Part model, mm, in its own coordinate system. Round coordinates to 2 decimals unless told otherwise and drop trailing zeros. Loops run counter-clockwise (first coordinate to the right, second up) from the corner with the lowest first, then second, coordinate; pieces in that order, holes last. Notation, with made-up numbers: (-19.5, 60) - (23.5, 60) arc R11 cw to (23.5, 79) - close; hole circle Ø9 at (8.25, 29). An arc over 180 degrees is marked (long way). Write each question's results on one line, items separated by ' | '. Start each with the question number.
(1) Cut at A-A, the plane z = 288. List the corners of the cut face in (x, y) (3 decimals).
(2) Cut at B-B, the plane x = -4. List the corners of the cut face in (y, z) (3 decimals).
(3) Flat gauge pin, fed straight in: P1, Ø4, axis at y = 25.4, z = 25.4, coming from the +X side. Where does the tip first touch, or does it go through?
(4) Drill centre lines: L1, parallel to Y at x = 10.65, z = 25.4; L2, parallel to X at y = 15, z = 79.5 (3 decimals); L3, parallel to Y at x = 4.25, z = 391.5 (3 decimals). Where is each one in solid material? Low to high.
Autodesk Inventor part; units mm, degrees
ref_plane "Start Plane" through (0, 0, -12.7) normal (0, 0, 1) x (1, 0, 0)
ref_plane "End Plane" through (0, 0, 749.3) normal (0, 0, 1) x (1, 0, 0)
ref_plane "Work Plane6" through (609.6, 0, -12.7) normal (0, 0, -1) x (-1, 0, 0)
ref_plane "Start Plane" through (0, 0, -12.7) normal (0, 0, 1) x (1, 0, 0)
ref_plane "End Plane" through (0, 0, 749.3) normal (0, 0, 1) x (1, 0, 0)
sketch "Sketch" plane through (0, 0, 0) normal (0, 0, 1) x (1, 0, 0)
  line L0 (-12.7, -38.1) -> (12.7, -38.1)
  line L1 (12.7, -38.1) -> (12.7, 38.1)
  line L2 (12.7, 38.1) -> (-12.7, 38.1)
  line L3 (-12.7, 38.1) -> (-12.7, -38.1)
  line L4 (-12.7, -38.1) -> (12.7, 38.1) construction
  line L5 (12.7, -38.1) -> (-12.7, 38.1) construction
  line L6 (-9.525, -34.925) -> (9.525, -34.925)
  line L7 (9.525, -34.925) -> (9.525, 34.925)
  line L8 (9.525, 34.925) -> (-9.525, 34.925)
  line L9 (-9.525, 34.925) -> (-9.525, -34.925)
  line L10 (-9.525, -34.925) -> (9.525, 34.925) construction
  line L11 (9.525, -34.925) -> (-9.525, 34.925) construction
  point P0 (0, 0)
  dimension "d0" = 25.4
  dimension "d1" = 76.2
  dimension "d2" = 3.175
  dimension "d3" = 3.175
extrude "Body" add sketch "Sketch" along normal up to surface (762 mm away) from surface at -12.7
sketch "Sketch6" plane through (0, 0, 0) normal (0, 0, 1) x (1, 0, 0)
  line L0 (0, 0) -> (10, 0)
ref_plane "Work Plane5" through (0, 0, 0) normal (0, -1, 0) x (1, 0, 0)
sketch "Sketch7" plane through (0, 0, 0) normal (0, -1, 0) x (1, 0, 0)
  line L0 (-2, -12.7) -> (12, -12.7)
  line L1 (-2, 749.3) -> (12, 749.3)
  dimension "d11" = 762
ref_plane "Work Plane6" through (609.6, 0, -12.7) normal (0, 0, -1) x (-1, 0, 0)
split "Split1" plane through (609.6, 0, -12.7) removes the side toward (0, 0, -1)
ref_plane "Work Plane7" through (0, 38.1, 749.3) normal (0, 0, 1) x (1, 0, 0)
split "Split2" plane through (0, 38.1, 749.3) removes the side toward (0, 0, 1)
sketch "Sketch8" plane through (-12.7, -38.1, 749.3) normal (-1, 0, 0) x (0, 0, 1)
  circle A0 centre (-381, 28.575) radius 14.2875
  line L0 (-762, 0) -> (0, 0)
  line L1 (-762, 76.2) -> (-762, 0)
  line L2 (0, 76.2) -> (-762, 76.2)
  line L3 (-622.3, 31.75) -> (-711.2, 31.75) construction
  line L4 (-622.3, 23.7871) -> (-711.2, 23.7871)
  line L5 (-711.2, 39.7129) -> (-622.3, 39.7129)
  arc A1 (-622.3, 23.7871) -> (-622.3, 39.7129) centre (-622.3, 31.75) ccw
  arc A2 (-711.2, 39.7129) -> (-711.2, 23.7871) centre (-711.2, 31.75) ccw
  line L6 (-139.7, 31.75) -> (-50.8, 31.75) construction
  line L7 (-139.7, 23.7871) -> (-50.8, 23.7871)
  line L8 (-50.8, 39.7129) -> (-139.7, 39.7129)
  arc A3 (-139.7, 39.7129) -> (-139.7, 23.7871) centre (-139.7, 31.75) ccw
  arc A4 (-50.8, 23.7871) -> (-50.8, 39.7129) centre (-50.8, 31.75) ccw
  line L9 (0, 0) -> (0, 76.2)
  line L10 (-381, 76.2) -> (-381, 0) construction
  line L11 (-762, 0) -> (0, 0) construction
  point P0 (-762, 73.025)
  point P1 (-666.75, 31.75)
  point P2 (-95.25, 31.75)
  dimension "d16" = 28.575
  dimension "d44" = 7.9629
  dimension "d45" = 7.9629
  dimension "d46" = 88.9
  dimension "d47" = 88.9
  dimension "d48" = 50.8
  dimension "d49" = 50.8
  dimension "d50" = 31.75
  dimension "d51" = 31.75
  dimension "d52" = 28.575
extrude "Extrusion3" cut sketch "Sketch8" against normal blind 25.4 contours A0 | L4 A2 L5 A1 | A3 L8 A4 L7
sketch "Sketch9" plane through (12.7, -38.1, 749.3) normal (1, 0, 0) x (0, 0, -1)
  line L0 (762, 76.2) -> (0, 76.2)
  line L1 (0, 76.2) -> (0, 0)
  point P0 (749.3, 38.1)
  point P1 (12.7, 63.5)
  point P2 (723.9, 63.5)
  point P3 (12.7, 12.7)
  point P4 (723.9, 12.7)
  dimension "d21" = 12.7
  dimension "d22" = 12.7
  dimension "d25" = 711.2
  dimension "d28" = 50.8
hole "Hole1" at (12.7, 25.4, 736.6) at (12.7, 25.4, 25.4) at (12.7, -25.4, 736.6) at (12.7, -25.4, 25.4) direction (-1, 0, 0) diameter 4.9784 end through all
equation "\"d0\" = Width"
equation "\"d1\" = Height"
equation "\"d2\" = Thickness"
equation "\"d3\" = Thickness"
equation "\"d45\" = d44"
equation "\"d47\" = d46"
equation "\"d49\" = d48"
equation "\"d51\" = d50"
equation "\"Height\" = 76.2"
equation "\"Width\" = 25.4"
equation "\"Thickness\" = 3.175"
equation "\"BaseLength\" = 736.6"
equation "\"G_OFFSET_START\" = 12.7"
equation "\"G_OFFSET_END\" = 12.7"
equation "\"d6\" = -G_OFFSET_START"
equation "\"d7\" = BaseLength + G_OFFSET_END"
equation "\"G_L\" = d11"
properties part number "AL RECT TUBE 3 x 1 x 0.125" material "Aluminum 6061"
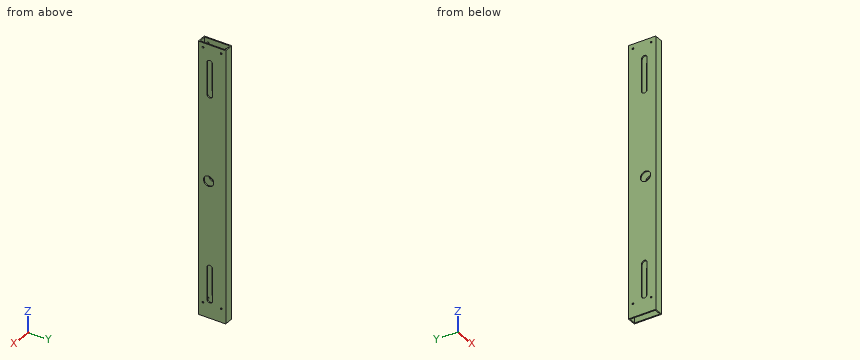
A:
1) outline: (-12.7, -38.1) - (12.7, -38.1) - (12.7, 38.1) - (-12.7, 38.1) - close; hole (-9.525, -34.925) - (9.525, -34.925) - (9.525, 34.925) - (-9.525, 34.925) - close
2) outline: (-38.1, -12.7) - (-34.925, -12.7) - (-34.925, 749.3) - (-38.1, 749.3) - close; (34.925, -12.7) - (38.1, -12.7) - (38.1, 749.3) - (34.925, 749.3) - close
3) P1: through
4) L1: -38.1 to -27.89, -22.91 to 22.91, 27.89 to 38.1 | L2: -12.7 to -9.525, 9.525 to 12.7 | L3: -38.1 to -34.925, 34.925 to 38.1
